from build123d import *

# Parameters (mm, degrees)
SKETCH1_R             = 20
BOSS_EXTRUDE1_DEPTH   = 200
BOSS_EXTRUDE1_2_DEPTH = 200
BOSS_EXTRUDE1_3_DEPTH = 200
BOSS_EXTRUDE1_4_DEPTH = 200
SKETCH2_W             = 400
SKETCH2_H             = 400
SKETCH2_R             = 25
BOSS_EXTRUDE2_DEPTH   = 20
SKETCH3_R             = 40
SKETCH3_R_2           = 25
BOSS_EXTRUDE3_DEPTH   = 20


with BuildPart() as part:
    # Sketch1 → Boss-Extrude1 (new body)
    with BuildSketch(Plane(origin=(0, 0, 0), x_dir=(1, 0, 0), z_dir=(0, 1, 0))):
        with Locations((-143.431457505, 143.431457505)):
            Circle(SKETCH1_R)
    extrude(amount=BOSS_EXTRUDE1_DEPTH)



with BuildPart() as body_2:
    # Sketch1 → Boss-Extrude1 2 (new body)
    with BuildSketch(Plane(origin=(0, 0, 0), x_dir=(1, 0, 0), z_dir=(0, 1, 0))):
        with Locations((-143.431457505, -143.431457505)):
            Circle(SKETCH1_R)
    extrude(amount=BOSS_EXTRUDE1_2_DEPTH)


with BuildPart() as body_3:
    # Sketch1 → Boss-Extrude1 3 (new body)
    with BuildSketch(Plane(origin=(0, 0, 0), x_dir=(1, 0, 0), z_dir=(0, 1, 0))):
        with Locations((143.431457505, -143.431457505)):
            Circle(SKETCH1_R)
    extrude(amount=BOSS_EXTRUDE1_3_DEPTH)


with BuildPart() as body_4:
    # Sketch1 → Boss-Extrude1 4 (new body)
    with BuildSketch(Plane(origin=(0, 0, 0), x_dir=(1, 0, 0), z_dir=(0, 1, 0))):
        with Locations((143.431457505, 143.431457505)):
            Circle(SKETCH1_R)
    extrude(amount=BOSS_EXTRUDE1_4_DEPTH)


with BuildPart() as part_1:
    add(part.part)

    add(body_2.part)  # Boss-Extrude2 merges body 2

    add(body_3.part)  # Boss-Extrude2 merges body 3

    add(body_4.part)  # Boss-Extrude2 merges body 4
    # Sketch2 → Boss-Extrude2 (add)
    with BuildSketch(Plane(origin=(0, 200, 0), x_dir=(1, 0, 0), z_dir=(0, 1, 0))):
        Rectangle(SKETCH2_W, SKETCH2_H)
        Circle(SKETCH2_R, mode=Mode.SUBTRACT)
    extrude(amount=BOSS_EXTRUDE2_DEPTH)

    # Sketch3 → Boss-Extrude3 (add)
    with BuildSketch(Plane(origin=(0, 220, 0), x_dir=(1, 0, 0), z_dir=(0, 1, 0))):
        Circle(SKETCH3_R)
        Circle(SKETCH3_R_2, mode=Mode.SUBTRACT)
    extrude(amount=BOSS_EXTRUDE3_DEPTH)


solid = part_1.part
Geometry check sheet. Reference: the model listing, model coordinates, mm. A direction names the side the tool comes from. Round coordinates to 2 decimals unless told otherwise and drop trailing zeros. Loops run counter-clockwise (first coordinate to the right, second up) from the corner with the lowest first, then second, coordinate; pieces in that order, holes last. Notation, with made-up numbers: (72, 46) -> (124, 46) arc R28 cw to (124, 80) -> close; hole circle Ø7 at (6, 83). An arc over 180 degrees is marked (long way). Answer as a JSON object with one key per item and string values. Group by question number.
Item 1: Release check for a two-part mould opening along Z. For faces 4 (the face through (23.846, 219.72, -7.509)), 5 (the face through (-3, 210, -200)), 6 (the face through (-144, 0, 143)), 7 (the face through (-3, 210, 200)) record: pulls with the +Z half, pulls with the -Z half, needs draft (parallel to the pull), parting line crosses it, or undercut.
Item 2: Cross-section at D-D, the plane x = -109.5. Record the cut outline in (y, z), plus the area to 3 significant figures.
Item 3: Thickness scan on line 1 along Z through (x, y) = (-144.5, 147); line 2 along X through (y, z) = (230.5, 0). Record the ranges inside material, lowest first.
Item 4: Cross-section at C-C, the plane y = 132.5. Record the cut outline in (x, z), plus the area to 3 significant figures.
Item 5: Cross-section at B-B, the plane x = 0. Record the cut outline in (y, z).
Item 6: Cross-section at A-A, the plane z = 0. Record the cut outline in (x, y), plus the area to 3 significant figures.
Item 7: Depth check by flat-ended pin: pin 1 Ø2 at (x, z) = (-64, 63) entering from -Y; pin 2 Ø2 at (x, z) = (9.5, -79.5) entering from +Y. Enter the tip coordinate at first touch or a pass-through.
Item 8: Set-up check for faces 1 (the face through (17.22, 240, -18.34)), 2 (the face through (-124.957, 98.6, 151.092)), 3 (the face through (-8.67, 229.86, 39.05)): record each of +Z, -Z, +X, -X, +Y, -Y from which the full face is reachable in a straight line by a thin tool's end or side.
Determined:
{
 "1": {"face 4": "undercut", "face 5": "pulls with the -Z half", "face 6": "needs draft", "face 7": "pulls with the +Z half"},
 "2": {"outline": "(200, -200) -> (220, -200) -> (220, 200) -> (200, 200) -> close", "area": "8,000 mm²"},
 "3": {"line 1": "z = -163.4 to -123.46, 123.46 to 163.4", "line 2": "x = -40 to -25, 25 to 40"},
 "4": {"outline": "circle Ø40 at (-143.43, -143.43); circle Ø40 at (-143.43, 143.43); circle Ø40 at (143.43, -143.43); circle Ø40 at (143.43, 143.43)", "area": "5,030 mm²"},
 "5": {"outline": "(200, -200) -> (220, -200) -> (220, -40) -> (240, -40) -> (240, -25) -> (200, -25) -> close; (200, 25) -> (240, 25) -> (240, 40) -> (220, 40) -> (220, 200) -> (200, 200) -> close"},
 "6": {"outline": "(-200, 200) -> (-25, 200) -> (-25, 240) -> (-40, 240) -> (-40, 220) -> (-200, 220) -> close; (25, 200) -> (200, 200) -> (200, 220) -> (40, 220) -> (40, 240) -> (25, 240) -> close", "area": "7,600 mm²"},
 "7": {"pin 1": "stops at y = 200", "pin 2": "stops at y = 220"},
 "8": {"face 1": "+Z, -Z, +X, -X, +Y", "face 2": "-Y", "face 3": "+Y"}
}
